from build123d import *

# Parameters (mm, degrees)
BOSS_EXTRUDE1_DEPTH = 400
BOSS_EXTRUDE2_DEPTH = 10
SKETCH3_R           = 43.000999871
CUT_EXTRUDE1_DEPTH  = 447.360216168
BOSS_EXTRUDE3_DEPTH = 7
SKETCH5_R           = 1.75
CUT_EXTRUDE2_DEPTH  = 33
SKETCH6_W           = 36.000000185
SKETCH6_H           = 60
BOSS_EXTRUDE4_DEPTH = 5
SKETCH7_W           = 7.24997928
SKETCH7_H           = 16
BOSS_EXTRUDE5_DEPTH = 53
SKETCH8_W           = 12.24997928
SKETCH8_H           = 60
BOSS_EXTRUDE6_DEPTH = 5
FILLET1_R           = 5
SKETCH10_W          = 20.000000185
SKETCH10_H          = 40
BOSS_EXTRUDE7_DEPTH = 7.24997928
CUT_EXTRUDE3_DEPTH  = 6
CUT_EXTRUDE4_DEPTH  = 68.845857758
SKETCH12_R          = 4.5
CUT_EXTRUDE5_DEPTH  = 16
CHAMFER2_SIZE       = 5
CHAMFER3_SIZE       = 5
SKETCH13_R          = 6.5
SKETCH13_R_2        = 4.5
BOSS_EXTRUDE8_DEPTH = 1
FILLET2_R           = 1


with BuildPart() as part:
    # Sketch1 → Boss-Extrude1 (new body)
    with BuildSketch(Plane(origin=(0, 200, 0), x_dir=(1, 0, 0), z_dir=(0, 1, 0))):
        with BuildLine():
            Line((1e-09, -3.855700002), (0.25, -4.00003757))
            Line((0.25, -4.00003757), (9.078700232, -4.00003757))
            ThreePointArc((9.078700232, -4.00003757), (9.652725366, -4.114218268), (10.139360377, -4.439377387))
            Line((10.139360377, -4.439377387), (12.500020747, -6.800037757))
            Line((12.500020747, -6.800037757), (12.500020747, -9.500037757))
            Line((12.500020747, -9.500037757), (13.00002072, -10.000037755))
            Line((13.00002072, -10.000037755), (17.00002072, -10.000037755))
            Line((17.00002072, -10.000037755), (17.500020747, -9.500037752))
            Line((17.500020747, -9.500037752), (17.500020747, -5.500037752))
            Line((17.500020747, -5.500037752), (17.00002075, -5.0000377))
            Line((17.00002075, -5.0000377), (14.30002072, -5.0000377))
            Line((14.30002072, -5.0000377), (14.085807141, -4.785824121))
            ThreePointArc((14.085807141, -4.785824121), (13.652261651, -4.136977442), (13.50002072, -3.371610598))
            Line((13.50002072, -3.371610598), (13.50002072, -0.30003757))
            Line((13.50002072, -0.30003757), (13.20002072, -3.757e-05))
            Line((13.20002072, -3.757e-05), (7.50002072, -3.757e-05))
            Line((7.50002072, -3.757e-05), (7.40002072, -0.10003757))
            Line((7.40002072, -0.10003757), (-7.40002072, -0.10003757))
            Line((-7.40002072, -0.10003757), (-7.50002072, -3.757e-05))
            Line((-7.50002072, -3.757e-05), (-13.20002072, -3.757e-05))
            Line((-13.20002072, -3.757e-05), (-13.50002072, -0.30003757))
            Line((-13.50002072, -0.30003757), (-13.50002072, -3.371610628))
            ThreePointArc((-13.50002072, -3.371610628), (-13.652261651, -4.136977472), (-14.085807141, -4.785824151))
            Line((-14.085807141, -4.785824151), (-14.30002069, -5.0000377))
            Line((-14.30002069, -5.0000377), (-17.00002072, -5.0000377))
            Line((-17.00002072, -5.0000377), (-17.50002072, -5.50003767))
            Line((-17.50002072, -5.50003767), (-17.50002072, -9.50003767))
            Line((-17.50002072, -9.50003767), (-17.000020665, -10.000037755))
            Line((-17.000020665, -10.000037755), (-13.00002072, -10.000037755))
            Line((-13.00002072, -10.000037755), (-12.500020741, -9.500037764))
            Line((-12.500020741, -9.500037764), (-12.500020741, -6.800037764))
            Line((-12.500020741, -6.800037764), (-10.139360364, -4.439377387))
            ThreePointArc((-10.139360364, -4.439377387), (-9.652725352, -4.114218268), (-9.078700218, -4.00003757))
            Line((-9.078700218, -4.00003757), (-0.25, -4.00003757))
            Line((-0.25, -4.00003757), (1e-09, -3.855700002))
        make_face()
    extrude(amount=-BOSS_EXTRUDE1_DEPTH)

    # Sketch3 → Cut-Extrude1 (cut)
    with BuildSketch(Plane(origin=(0, 200, 0), x_dir=(1, 0, 0), z_dir=(0, 1, 0))):
        with Locations((0, -0.10003757)):
            Circle(SKETCH3_R)
    extrude(amount=-CUT_EXTRUDE1_DEPTH, mode=Mode.SUBTRACT)


with BuildPart() as body_2:
    # Sketch2 → Boss-Extrude2 (new body)
    with BuildSketch(Plane(origin=(0, 210, 0), x_dir=(1, 0, 0), z_dir=(0, 1, 0))):
        Polygon((-8.353826469, -7.25003757), (8.353826482, -7.25003757), (9.250020747, -8.146231835), (9.250020747, -10.846231788), (11.653826595, -13.250037755), (18.34621475, -13.250037755), (20.750020747, -10.846231878), (20.750020747, -4.153843779), (18.346214932, -1.7500377), (16.75002072, -1.7500377), (16.75002072, 1.046156508), (14.546214798, 3.24996243), (-14.546214798, 3.24996243), (-16.75002072, 1.046156508), (-16.75002072, -1.7500377), (-18.346214741, -1.7500377), (-20.75002072, -4.153843535), (-20.75002072, -10.846231691), (-18.3462148, -13.250037755), (-11.653826621, -13.250037755), (-9.250020741, -10.846231821), (-9.250020741, -8.146231842), align=None)
        with BuildLine():
            Line((13.303574111, 0.24996243), (-13.303574111, 0.24996243))
            Line((-13.303574111, 0.24996243), (-13.75002072, -0.196484179))
            Line((-13.75002072, -0.196484179), (-13.75002072, -3.371610628))
            ThreePointArc((-13.75002072, -3.371610628), (-13.883231534, -4.041306614), (-14.262583837, -4.609047456))
            Line((-14.262583837, -4.609047456), (-14.403574081, -4.7500377))
            Line((-14.403574081, -4.7500377), (-17.103574106, -4.7500377))
            Line((-17.103574106, -4.7500377), (-17.75002072, -5.396484275))
            Line((-17.75002072, -5.396484275), (-17.75002072, -9.603591056))
            Line((-17.75002072, -9.603591056), (-17.10357406, -10.250037755))
            Line((-17.10357406, -10.250037755), (-12.896467328, -10.250037755))
            Line((-12.896467328, -10.250037755), (-12.250020741, -9.603591153))
            Line((-12.250020741, -9.603591153), (-12.250020741, -6.903591155))
            Line((-12.250020741, -6.903591155), (-9.962583668, -4.616154083))
            ThreePointArc((-9.962583668, -4.616154083), (-9.557054494, -4.345188152), (-9.078700218, -4.25003757))
            Line((-9.078700218, -4.25003757), (9.078700232, -4.25003757))
            ThreePointArc((9.078700232, -4.25003757), (9.557054508, -4.345188152), (9.962583682, -4.616154083))
            Line((9.962583682, -4.616154083), (12.250020747, -6.903591148))
            Line((12.250020747, -6.903591148), (12.250020747, -9.603591144))
            Line((12.250020747, -9.603591144), (12.896467326, -10.250037755))
            Line((12.896467326, -10.250037755), (17.103574107, -10.250037755))
            Line((17.103574107, -10.250037755), (17.750020747, -9.603591147))
            Line((17.750020747, -9.603591147), (17.750020747, -5.39648437))
            Line((17.750020747, -5.39648437), (17.103574149, -4.7500377))
            Line((17.103574149, -4.7500377), (14.403574111, -4.7500377))
            Line((14.403574111, -4.7500377), (14.262583837, -4.609047426))
            ThreePointArc((14.262583837, -4.609047426), (13.883231534, -4.041306584), (13.75002072, -3.371610598))
            Line((13.75002072, -3.371610598), (13.75002072, -0.196484179))
            Line((13.75002072, -0.196484179), (13.303574111, 0.24996243))
        make_face(mode=Mode.SUBTRACT)
    extrude(amount=BOSS_EXTRUDE2_DEPTH)

    # Sketch4 → Boss-Extrude3 (add)
    with BuildSketch(Plane(origin=(0, 210, 0), x_dir=(-1, 0, 0), z_dir=(0, -1, 0))):
        Polygon((27, -13.250037755), (27, 22.74996243), (-27, 22.74996243), (-27, -13.250037755), (-18.34621475, -13.250037755), (-20.750020747, -10.846231878), (-20.750020747, -4.153843779), (-18.346214932, -1.7500377), (-16.75002072, -1.7500377), (-16.75002072, 1.046156508), (-14.546214798, 3.24996243), (14.546214798, 3.24996243), (16.75002072, 1.046156508), (16.75002072, -1.7500377), (18.346214741, -1.7500377), (20.75002072, -4.153843535), (20.75002072, -10.846231691), (18.3462148, -13.250037755), align=None)
    extrude(amount=-BOSS_EXTRUDE3_DEPTH)

    # Sketch5 → Cut-Extrude2 (cut)
    with BuildSketch(Plane(origin=(0, 210, 0), x_dir=(-1, 0, 0), z_dir=(0, -1, 0))):
        with Locations(Location((22.5, 18.24996243, 0), (0, 0, 90))):
            Circle(SKETCH5_R)
        with Locations(Location((22.5, 8.24996243, 0), (0, 0, 90))):
            Circle(SKETCH5_R)
        with Locations(Location((-22.5, 8.24996243, 0), (0, 0, 90))):
            Circle(SKETCH5_R)
        with Locations(Location((-22.5, 18.24996243, 0), (0, 0, 90))):
            Circle(SKETCH5_R)
    extrude(amount=-CUT_EXTRUDE2_DEPTH, mode=Mode.SUBTRACT)

    # Sketch6 → Boss-Extrude4 (add)
    with BuildSketch(Plane.ZY.offset(27)):
        with Locations((-4.749962337, 240)):
            Rectangle(SKETCH6_W, SKETCH6_H)
    extrude(amount=BOSS_EXTRUDE4_DEPTH)

    # Sketch7 → Boss-Extrude5 (add)
    with BuildSketch(Plane(origin=(0, 217, 0), x_dir=(1, 0, 0), z_dir=(0, 1, 0))):
        with Locations((-23.37501036, -5.250037755)):
            Rectangle(SKETCH7_W, SKETCH7_H)
    extrude(amount=BOSS_EXTRUDE5_DEPTH)

    # Sketch8 → Boss-Extrude6 (add)
    with BuildSketch(Plane(origin=(0, 0, -22.74996243), x_dir=(-1, 0, 0), z_dir=(0, 0, -1))):
        with Locations((25.87501036, 240)):
            Rectangle(SKETCH8_W, SKETCH8_H)
    extrude(amount=BOSS_EXTRUDE6_DEPTH)

    # Fillet1
    fillet1_edges = [body_2.edges().sort_by_distance(p)[0] for p in [
        (-19.75002072, 213.5, -22.74996243),
    ]]
    fillet(fillet1_edges, radius=FILLET1_R - 0.0001)  # a hair under: the kernel refuses the full size

    # Sketch10 → Boss-Extrude7 (add)
    with BuildSketch(Plane(origin=(-27, 0, 0), x_dir=(0, 0, -1), z_dir=(1, 0, 0))):
        with Locations((12.749962337, 250)):
            Rectangle(SKETCH10_W, SKETCH10_H)
    extrude(amount=BOSS_EXTRUDE7_DEPTH)

    # Sketch9 → Cut-Extrude3 (cut)
    with BuildSketch(Plane(origin=(-19.75002072, 0, 0), x_dir=(0, 0, -1), z_dir=(1, 0, 0))):
        Polygon((14.755515837, 250), (11.002739087, 256.5), (3.497185588, 256.5), (-0.255591162, 250), (3.497185588, 243.5), (11.002739087, 243.5), align=None)
    extrude(amount=-CUT_EXTRUDE3_DEPTH, mode=Mode.SUBTRACT)

    # Sketch11 → Cut-Extrude4 (cut, through all)
    with BuildSketch(Plane(origin=(0, 217, 0), x_dir=(1, 0, 0), z_dir=(0, 1, 0))):
        with BuildLine():
            Line((-22.5, 20.74996243), (-17.824832595, 20.74996243))
            Line((-17.824832595, 20.74996243), (-17.824832595, 15.74996243))
            Line((-17.824832595, 15.74996243), (-22.5, 15.74996243))
            ThreePointArc((-22.5, 15.74996243), (-25, 18.24996243), (-22.5, 20.74996243))
        make_face()
        with BuildLine():
            Line((-22.5, 10.74996243), (-17.824832595, 10.74996243))
            Line((-17.824832595, 10.74996243), (-17.824832595, 5.74996243))
            Line((-17.824832595, 5.74996243), (-22.5, 5.74996243))
            ThreePointArc((-22.5, 5.74996243), (-25, 8.24996243), (-22.5, 10.74996243))
        make_face()
    extrude(amount=CUT_EXTRUDE4_DEPTH, mode=Mode.SUBTRACT)

    # Sketch12 → Cut-Extrude5 (cut)
    with BuildSketch(Plane(origin=(-25.75002072, 0, 0), x_dir=(0, 0, -1), z_dir=(1, 0, 0))):
        with Locations((7.249962338, 250)):
            Circle(SKETCH12_R)
    extrude(amount=-CUT_EXTRUDE5_DEPTH, mode=Mode.SUBTRACT)

    # Chamfer2
    chamfer2_edges = [body_2.edges().sort_by_distance(p)[0] for p in [
        (-32, 270, -7.249962337),
    ]]
    chamfer(chamfer2_edges, length=CHAMFER2_SIZE)

    # Chamfer3
    chamfer3_edges = [body_2.edges().sort_by_distance(p)[0] for p in [
        (-32, 210, -7.249962338),
    ]]
    chamfer(chamfer3_edges, length=CHAMFER3_SIZE)

    # Sketch13 → Boss-Extrude8 (add)
    with BuildSketch(Plane.ZY.offset(32)):
        with Locations(Location((-7.249962338, 250, 0), (0, 0, 180))):
            Circle(SKETCH13_R)
        with Locations(Location((-7.249962338, 250, 0), (0, 0, 180))):
            Circle(SKETCH13_R_2, mode=Mode.SUBTRACT)
    extrude(amount=BOSS_EXTRUDE8_DEPTH)

    # Fillet2
    fillet2_edges = [body_2.edges().sort_by_distance(p)[0] for p in [
        (-32, 250, -0.749962338),
    ]]
    fillet(fillet2_edges, radius=FILLET2_R - 0.0001)  # a hair under: the kernel refuses the full size


solid = body_2.part
Can you work these out from the model? Positions are in its coordinate system, mm. A direction names the side the tool comes from. Round coordinates to 2 decimals unless told otherwise and drop trailing zeros. Order: outer loops, then holes, each group sorted by start corner. A loop starts at its lowest first (then second) coordinate and runs counter-clockwise, first axis right, second up. Notation, with made-up numbers: (2, 44.25) - (29, 44.25) arc R30 ccw to (29, 67.25) - close; hole circle Ø1 at (70, 56.25). An arc over 180 degrees is marked (long way). Answer in a Markdown table with one row per item.
(1) Suppose I cut it at B-B, the plane z = -17.5. Please give me the cut outline in (x, y), plus the area to 3 significant figures.
From the geometry:
| item | result |
|---|---|
| outline | (-32, 215) - (-27, 210) - (-24.08, 210) - (-24.08, 217) - (-27, 217) - (-27, 230) - (-24.88, 230) - (-24.88, 270) - (-27, 270) - (-32, 265) - close; (-20.92, 210) - (20.92, 210) - (20.92, 217) - (-20.92, 217) - close; (24.08, 210) - (27, 210) - (27, 217) - (24.08, 217) - close |
| area | 693 mm2 |
(2) If we mould it in two halves opening along Z, with no side actions, what happens to faces 4 (the face through (-24, 240, 13.25)), 5 (the face through (-22.71, 246.7, -12.85)), 6 (the face through (-19.75, 244, 4))? For each: released by +Z, released by -Z, zero draft, split by the parting line, or undercut.
From the geometry:
| item | result |
|---|---|
| face 4 | released by +Z |
| face 5 | undercut |
| face 6 | zero draft |
(3) Suppose I cut it at A-A, the plane x = 22.5. Please give me the cut outline in (y, z).
From the geometry:
| item | result |
|---|---|
| outline | (210, -22.75) - (217, -22.75) - (217, -20) - (210, -20) - close; (210, -16.5) - (217, -16.5) - (217, -10) - (210, -10) - close; (210, -6.5) - (217, -6.5) - (217, 13.25) - (210, 13.25) - close |
(4) Suppose I cut it at D-D, the plane x = -28.5. Please give me the cut outline in (y, z).
From the geometry:
| item | result |
|---|---|
| outline | (211.5, -27.75) - (268.5, -27.75) - (268.5, 13.25) - (211.5, 13.25) - close; hole circle Ø9 at (250, -7.25) |
(5) Which directions (+Z, -Z, +X, -X, +Y, -Y) give clear straight access to the entire face, cutting with the end or side of a thin tool? Please do faces 1 (the face through (0, 215, 7.25)), 2 (the face through (17.75, 215, 8)), 3 (the face through (-21, 263, -5.75)).
From the geometry:
| item | result |
|---|---|
| face 1 | +Z, +Y, -Y |
| face 2 | +Y, -Y |
| face 3 | +X, +Y |
(6) Suppose I cut it at C-C, the plane y = 221. Please give me the cut outline in (x, z).
From the geometry:
| item | result |
|---|---|
| outline | (-32, -27.75) - (-19.75, -27.75) - (-19.75, -22.75) - (-27, -22.75) - (-27, -2.75) - (-19.75, -2.75) - (-19.75, 13.25) - (-32, 13.25) - close |
(7) Please list where these lines run through material, in increasing order: L1, parallel to Z at x = -24.5, y = 229.5; L2, parallel to Z at x = -22, y = 212; L3, parallel to Z at x = 17, y = 213. Write a range as from..to.
From the geometry:
| item | result |
|---|---|
| L1 | z = -27.75..-22.75, -2.75..13.25 |
| L2 | z = -27.75..-19.93, -16.57..-9.93, -6.57..13.25 |
| L3 | z = -22.75..4.75, 10.25..13.25 |
(8) For P1, Ø6, axis at y = 257, z = 5.5, coming from the +X side; P2, Ø8, axis at y = 221, z = -12.5, coming from the -X side; P3, Ø3.5, axis at x = 3.5, y = 219, coming from the -Z side, each with a flat end and sliding along its axis, tell me the tip position at first contact or that it passes through.
From the geometry:
| item | result |
|---|---|
| P1 | stops at x = -19.75 |
| P2 | stops at x = -32 |
| P3 | stops at z = -3.25 |
